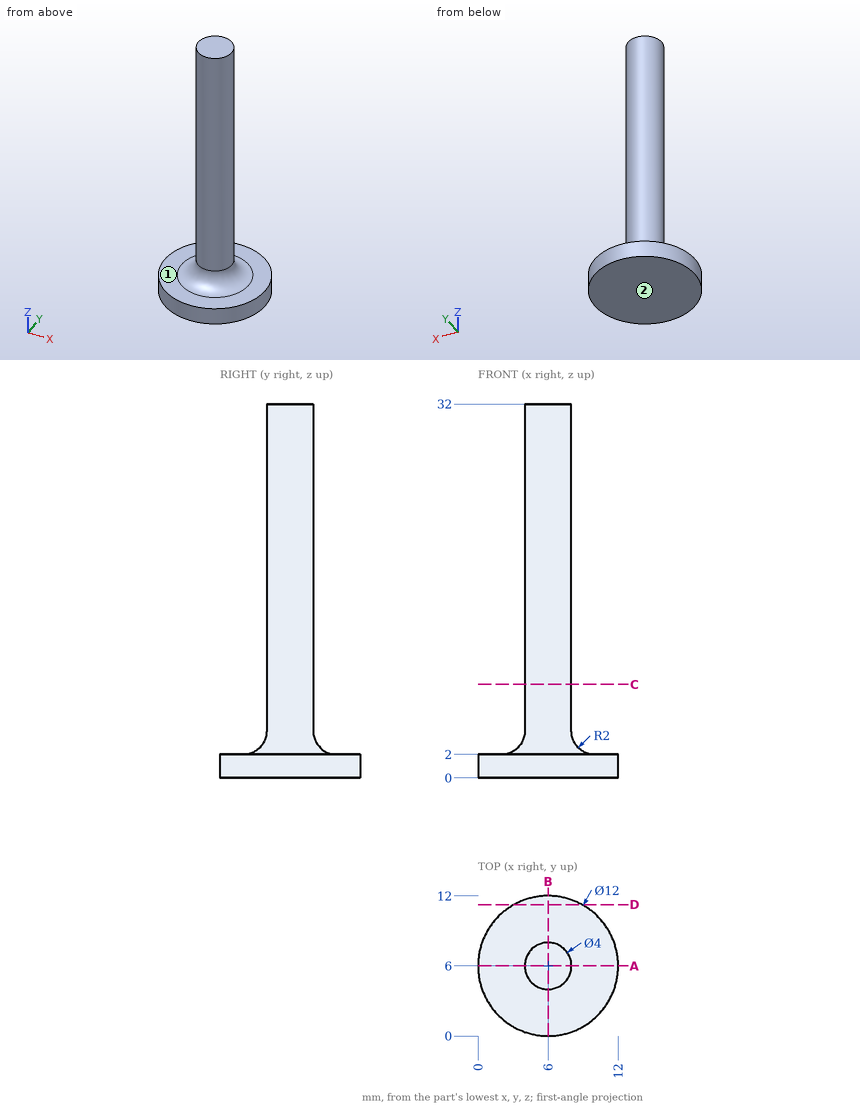
Design review of the part shown in the three views and the two pictorial views. Dimensions are in mm from the part's minimum x, y and z. A direction names the side the tool comes from. Give positions to 0.01 mm unless a question says otherwise; leave off trailing zeros. Loops run counter-clockwise (first coordinate to the right, second up) from the corner with the lowest first, then second, coordinate; pieces in that order, holes last. Notation, with made-up numbers: M 84.5,-6.5 L 138.5,-6.5 A30 ccw 138.5,25.5 Z; hole C 64,70.25 d9. An arc over 180 degrees is marked long. Put each result on its own line as item: value. Start each with the question number.
(1) Machinability: for the marked faces 1 and 2, which of the approach directions +Z, -Z, +X, -X, +Y, -Y give a long, thin tool a straight path to every point of the face, cutting with its end or side? Answer none if there is none.
(2) For pin 1 (5 mm diameter, centred on x = 6.5, z = 14, fed in from +Y); pin 2 (1.5 mm diameter, centred on x = 2.5, y = 4, fed in from +Z); pin 3 (1.5 mm diameter, centred on y = 8, z = 25, fed in from -X); pin 4 (6 mm diameter, centred on x = 8.5, y = 8, fed in from -Z), all flat-tipped, find the tip position at first contact; note any pin that passes through.
(3) Add section A-A, the plane y = 6. Write out the cut boundary in (x, z).
(4) Add section C-C, the plane z = 8. Write out the cut boundary in (x, y).
(5) Add section D-D, the plane y = 11.25. Write out the cut boundary in (x, z).
(6) Wall thickness on L1, parallel to Z at x = 2.25, y = 8.75; L2, parallel to Y at x = 6, z = 12; L3, parallel to Y at x = 5.5, z = 25: over which ranges is each line inside the solid? List them lowest first.
Result:
1. face 1: +Z
1. face 2: -Z, +X, -X, +Y, -Y
2. pin 1: stops at y = 8
2. pin 2: stops at z = 2.13
2. pin 3: stops at x = 4.44
2. pin 4: stops at z = 0
3. outline: M 0,0 L 12,0 L 12,2 L 10,2 A2 cw 8,4 L 8,32 L 4,32 L 4,4 A2 cw 2,2 L 0,2 Z
4. outline: C 6,6 d4
5. outline: M 3.1,0 L 8.9,0 L 8.9,2 L 3.1,2 Z
6. L1: z = 0 to 2
6. L2: y = 4 to 8
6. L3: y = 4.06 to 7.94
